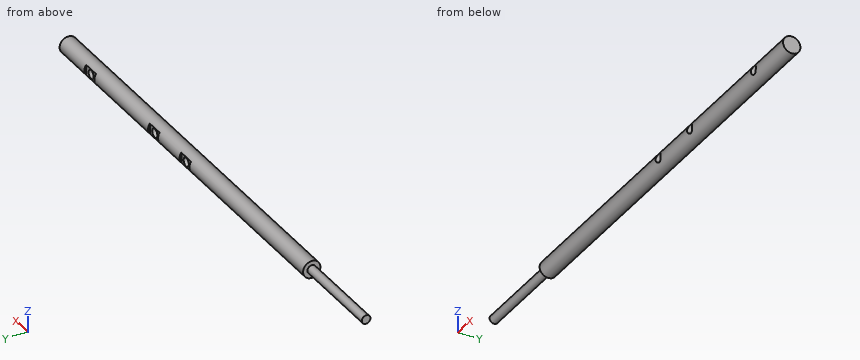
```python
from build123d import *

# Parameters (mm, degrees)
SKETCH2_R                        = 3.175
MAIN_SHAFT_DEPTH                 = 95.25
PIN_HOLES_CUT_DEPTH              = 96.355774602
PIN_HOLES_CUT_DEPTH_BACK         = 96.355774602
SKETCH3_R                        = 1.63195
FLAT_FOR_DRILLING_CUT_DEPTH      = 96.355774709
FLAT_FOR_DRILLING_CUT_DEPTH_BACK = 96.355774709
SKETCH5_W                        = 6.35
SKETCH5_H                        = 0.635
F_1_8_CUT_DEPTH                  = 191.552909422
F_1_8_CUT_DEPTH_BACK             = 34.75482
SKETCH6_R                        = 3.175
SKETCH6_R_2                      = 1.5875
CUT_EXTRUDE1_DEPTH               = 96.355774709
CUT_EXTRUDE1_DEPTH_BACK          = 96.355774709
SKETCH7_R                        = 1.6
CUT_EXTRUDE2_START               = 2.54
SKETCH7_3_W                      = 6.35
SKETCH7_3_H                      = 13.17395124
SKETCH7_3_R                      = 1.6
CUT_EXTRUDE2_DEPTH               = 93.815774709


with BuildPart() as part:
    # Sketch2 → Main Shaft (new, symmetric)
    with BuildSketch(Plane(origin=(0, 0, 0), x_dir=(0, 0, -1), z_dir=(1, 0, 0))):
        Circle(SKETCH2_R)
    extrude(amount=MAIN_SHAFT_DEPTH, both=True)

    # Sketch3 → Pin Holes Cut (cut, two sides: drawn at the far end of the back side and taken through both)
    with BuildSketch(Plane(origin=(0, 0, 0), x_dir=(1, 0, 0), z_dir=(0, 1, 0)).offset(-PIN_HOLES_CUT_DEPTH_BACK)):
        with Locations(Location((15.3416, 0, 0), (0, 0, 270))):
            Circle(SKETCH3_R)
        with Locations(Location((35.4584, 0, 0), (0, 0, 270))):
            Circle(SKETCH3_R)
    extrude(amount=PIN_HOLES_CUT_DEPTH + PIN_HOLES_CUT_DEPTH_BACK, mode=Mode.SUBTRACT)

    # Sketch5 → Flat for drilling Cut (cut, two sides: drawn at the far end of the back side and taken through both)
    with BuildSketch(Plane.XY.offset(-FLAT_FOR_DRILLING_CUT_DEPTH_BACK)):
        Polygon((18.5166, 3.175), (16.97355, 3.175), (13.70965, 3.175), (12.1666, 3.175), (12.1666, 2.54), (18.5166, 2.54), align=None)
        with Locations((35.45832639, 2.8575)):
            Rectangle(SKETCH5_W, SKETCH5_H)
    extrude(amount=FLAT_FOR_DRILLING_CUT_DEPTH + FLAT_FOR_DRILLING_CUT_DEPTH_BACK, mode=Mode.SUBTRACT)

    # Sketch6 → 1_8 Cut (cut, two sides: drawn at the far end of the back side and taken through both)
    with BuildSketch(Plane.ZY.offset(95.25).offset(-F_1_8_CUT_DEPTH_BACK)):
        Circle(SKETCH6_R)
        with Locations(Location((0, 0, 0), (0, 0, 180))):
            Circle(SKETCH6_R_2, mode=Mode.SUBTRACT)
    extrude(amount=F_1_8_CUT_DEPTH + F_1_8_CUT_DEPTH_BACK, mode=Mode.SUBTRACT)

    # Sketch7 → Cut-Extrude1 (cut, two sides: drawn at the far end of the back side and taken through both)
    with BuildSketch(Plane(origin=(0, 0, 0), x_dir=(1, 0, 0), z_dir=(0, 1, 0)).offset(-CUT_EXTRUDE1_DEPTH_BACK)):
        with Locations(Location((76.2, 0, 0), (0, 0, 270))):
            Circle(SKETCH7_R)
    extrude(amount=CUT_EXTRUDE1_DEPTH + CUT_EXTRUDE1_DEPTH_BACK, mode=Mode.SUBTRACT)

    # Sketch7_3 → Cut-Extrude2 (cut, through all)
    with BuildSketch(Plane(origin=(0, 0, 0), x_dir=(1, 0, 0), z_dir=(0, 1, 0)).offset(CUT_EXTRUDE2_START)):
        with Locations((76.2, 0)):
            Rectangle(SKETCH7_3_W, SKETCH7_3_H)
        with Locations(Location((76.2, 0, 0), (0, 0, 270))):
            Circle(SKETCH7_3_R, mode=Mode.SUBTRACT)
    extrude(amount=CUT_EXTRUDE2_DEPTH, mode=Mode.SUBTRACT)


solid = part.part
```
Geometry: final body of the model. Coordinates: model frame, mm. Round coordinates to 2 decimals unless told otherwise and drop trailing zeros. Write each loop counter-clockwise with the first axis right and the second up, starting at its lowest first coordinate (ties: lowest second). Pieces come first, ordered by that corner, then holes.
Item 1: Section query C-C (x = 76.2). Return loops of the section in (y, z) (3 decimals), plus the area to 3 significant figures.
Item 2: Section query D-D (x = 56). Return loops of the section in (y, z) (3 decimals), plus the area to 3 significant figures.
Item 3: Section query A-A (z = 0). Give the number of separate pieces and of enclosed holes in the cut face, plus the area to 3 significant figures.
Item 4: Material intervals for L1, parallel to X at y = -0.4, z = 0; L2, parallel to X at y = -2.5, z = -1; L3, parallel to Z at x = 61, y = 2.75, sorted ascending.
Item 5: Pin query (flat end, axial travel): P1, Ø1.1, axis at x = 74.5, z = -0.5, coming from the +Y side; P2, Ø0.5, axis at y = 3, z = 0, coming from the -X side. Return the tip coordinate at first contact, or that it passes through.
Completed:
1. outline: (-2.742, -1.6) arc R3.175 ccw to (2.54, -1.905) - (2.54, -1.6) - close; (-2.742, 1.6) - (2.54, 1.6) - (2.54, 1.905) arc R3.175 ccw to start
1. area: 12.2 mm2
2. outline: circle Ø6.35 at (0, 0)
2. area: 31.7 mm2
3. separate pieces: 4
3. enclosed holes: 0
3. area: 1,030 mm2
4. L1: x = -95.25 to 13.71, 16.97 to 33.83, 37.09 to 74.6, 77.8 to 95.25
4. L2: x = -60.5 to 14.05, 16.63 to 34.17, 36.75 to 74.95, 77.45 to 95.25
4. L3: z = -1.59 to 1.59
5. P1: stops at y = 2.54
5. P2: stops at x = -60.5
